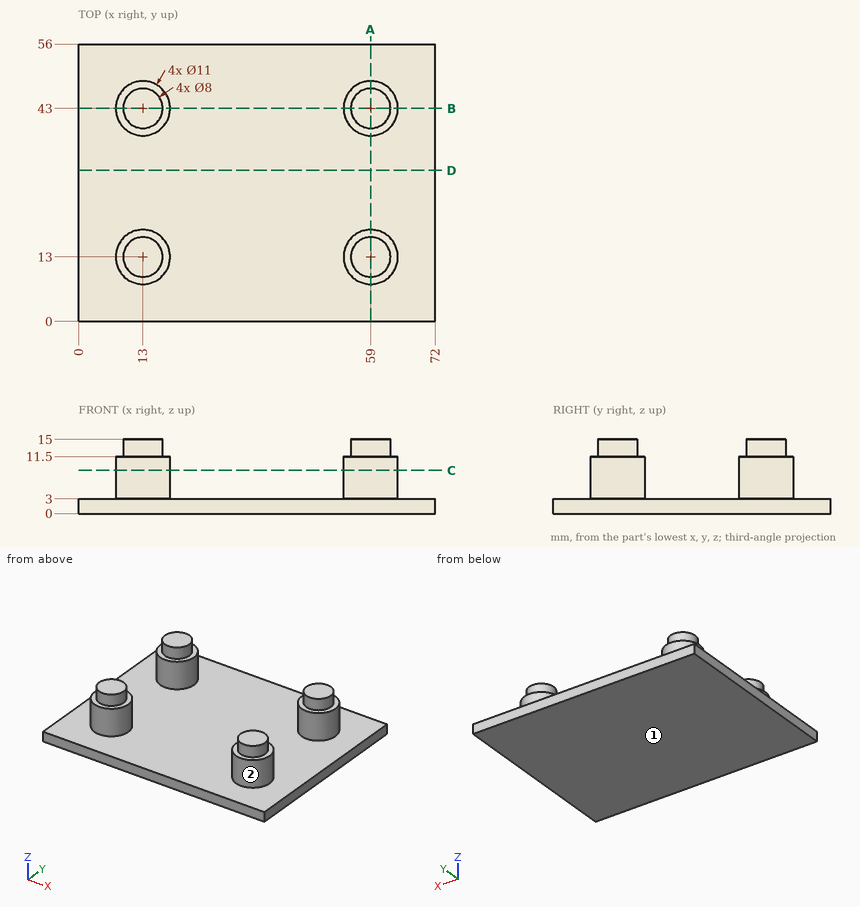
Study the drawing (mm; zero at the part's minimum x, y, z) and answer. Give positions to 0.01 mm unless a question says otherwise; leave off trailing zeros. Order: outer loops, then holes, each group sorted by start corner. A loop starts at its lowest first (then second) coordinate and runs counter-clockwise, first axis right, second up. Notation, with made-up numbers: (10, 39.25) - (26, 39.25) arc R36 ccw to (26, 74.25) - close; hole circle Ø2 at (34.5, -1.5). An arc over 180 degrees is marked (long way). Answer in a Markdown table with one row per item. Add a question column.
Q1. Given P1, Ø3, axis at y = 15, z = 13.5, coming from the -X side; P2, Ø3, axis at y = 8, z = 9, coming from the +X side; P3, Ø6, axis at y = 39, z = 7.5, coming from the -X side, each flat-ended and moving along its own axis, determine where each tip first touches the part or whether it passes through.
Q2. The part is cut by section C-C (z = 8.75). Determine the outline of the cut face in (x, y).
Q3. The part is cut by section A-A (x = 59). Determine the outline of the cut face in (y, z).
Q4. The part is cut by section B-B (y = 43). Determine the outline of the cut face in (x, z), then the cut area to 3 significant figures.
Q5. The part is cut by section D-D (y = 30.5). Determine the outline of the cut face in (x, z).
Q6. Find the intervals of material crossed by line 1 along Z through (x, y) = (18.5, 12); line 2 along Z through (x, y) = (16, 16); line 3 along X through (y, z) = (47, 9.75), in increasing order. Write a range as [from, to].
Q7. For a pull along Y with two mould halves and no side action, classify the marked faces 1 and 2 as released by +Y, released by -Y, zero draft, split by the parting line, or undercut.
Determined:
| question | item | result |
|---|---|---|
| 1 | P1 | stops at x = 9.03 |
| 1 | P2 | stops at x = 63.24 |
| 1 | P3 | stops at x = 7.59 |
| 2 | outline | circle Ø11 at (13, 13); circle Ø11 at (13, 43); circle Ø11 at (59, 13); circle Ø11 at (59, 43) |
| 3 | outline | (0, 0) - (56, 0) - (56, 3) - (48.5, 3) - (48.5, 11.5) - (47, 11.5) - (47, 15) - (39, 15) - (39, 11.5) - (37.5, 11.5) - (37.5, 3) - (18.5, 3) - (18.5, 11.5) - (17, 11.5) - (17, 15) - (9, 15) - (9, 11.5) - (7.5, 11.5) - (7.5, 3) - (0, 3) - close |
| 4 | outline | (0, 0) - (72, 0) - (72, 3) - (64.5, 3) - (64.5, 11.5) - (63, 11.5) - (63, 15) - (55, 15) - (55, 11.5) - (53.5, 11.5) - (53.5, 3) - (18.5, 3) - (18.5, 11.5) - (17, 11.5) - (17, 15) - (9, 15) - (9, 11.5) - (7.5, 11.5) - (7.5, 3) - (0, 3) - close |
| 4 | area | 459 mm² |
| 5 | outline | (0, 0) - (72, 0) - (72, 3) - (0, 3) - close |
| 6 | line 1 | z = [0, 3] |
| 6 | line 2 | z = [0, 11.5] |
| 6 | line 3 | x = [9.23, 16.77], [55.23, 62.77] |
| 7 | face 1 | zero draft |
| 7 | face 2 | undercut |
